```python
from build123d import *

# Parameters (mm, degrees)
F0_W     = 45
F0_H     = 45
F1_DEPTH = 3
F3_DEPTH = 25
F4_W     = 45
F4_H     = 45
F5_DEPTH = 5
F7_DEPTH = 25
F8_R     = 18
F9_DEPTH = 25


with BuildPart() as f1:
    # F0 (on Top) → F1 (new body)
    with BuildSketch(Plane.XY):
        Rectangle(F0_W, F0_H)
    extrude(amount=F1_DEPTH)

    # F2 (on face) → F3 (cut)
    with BuildSketch(Plane.XY.offset(3)):
        Polygon((11.5, 11.5), (-11.5, 11.5), (-11.5, 4), (-17.6846776158, 4), (-17.6846776158, -4), (-11.5, -4), (-11.5, -11.5), (11.5, -11.5), (11.5, -4), (17.6846776158, -4), (17.6846776158, 4), (11.5, 4), align=None)
    extrude(amount=-F3_DEPTH, mode=Mode.SUBTRACT)

    # F4 (on face) → F5 (join)
    with BuildSketch(Plane.XY.offset(3)):
        Rectangle(F4_W, F4_H)
    extrude(amount=F5_DEPTH)

    # F6 (on face) → F7 (cut)
    with BuildSketch(Plane(origin=(0, 0, 3), x_dir=(1, 0, 0), z_dir=(0, 0, -1))):
        Polygon((11.5, -11.5), (11.5, -4), (11.5, 4), (11.5, 11.5), (-11.5, 11.5), (-11.5, 4), (-11.5, -4), (-11.5, -11.5), align=None)
    extrude(amount=-F7_DEPTH, mode=Mode.SUBTRACT)

    # F8
    f8_edges = [f1.edges().sort_by_distance(p)[0] for p in [
        (-22.5, -22.5, 4),
        (22.5, -22.5, 4),
        (22.5, 22.5, 4),
        (-22.5, 22.5, 4),
    ]]
    fillet(f8_edges, radius=F8_R)

    # F9 (add): a face of the model
    f9_faces = [f1.faces().sort_by_distance(p)[0] for p in [
        (0, 21.8636038969, 8),
    ]]
    extrude(f9_faces, amount=F9_DEPTH)


solid = f1.part
```
Part model, mm, in its own coordinate system. A direction names the side the tool comes from. Round coordinates to 2 decimals unless told otherwise and drop trailing zeros. Write each loop counter-clockwise with the first axis right and the second up, starting at its lowest first coordinate (ties: lowest second). Pieces come first, ordered by that corner, then holes.
Item 1: Cut at D-D, the plane x = 17. Give the cut face in (y, z), plus the area to 3 significant figures.
Results:
outline: (-17.45, 0) - (-4, 0) - (-4, 3) - (4, 3) - (4, 0) - (17.45, 0) - (17.45, 33) - (-17.45, 33) - close
area: 1,130 mm2
Item 2: Which spindle directions (+Z, -Z, +X, -X, +Y, -Y) get a long thin tool onto all of the face, cutting with end or side? Do faces 4 (the flat face through (0, -15, 0)), 5 (the flat face through (-15, 0, 3)). Say none if no direction does.
Results:
face 4: -Z, +X, -X, +Y, -Y
face 5: -Z
Item 3: Cut at A-A, the plane x = -2.5. Give the cut face in (y, z), plus the area to 3 significant figures.
Results:
outline: (-22.5, 0) - (-11.5, 0) - (-11.5, 33) - (-22.5, 33) - close; (11.5, 0) - (22.5, 0) - (22.5, 33) - (11.5, 33) - close
area: 726 mm2
Item 4: Cut at B-B, the plane y = -1.5. Give the cut face in (x, z).
Results:
outline: (-22.5, 0) - (-17.68, 0) - (-17.68, 3) - (-11.5, 3) - (-11.5, 33) - (-22.5, 33) - close; (11.5, 3) - (17.68, 3) - (17.68, 0) - (22.5, 0) - (22.5, 33) - (11.5, 33) - close
Item 5: Cut at C-C, the plane z = 14. Give the cut face in (x, y).
Results:
outline: (-22.5, -4.5) arc R18 ccw to (-4.5, -22.5) - (4.5, -22.5) arc R18 ccw to (22.5, -4.5) - (22.5, 4.5) arc R18 ccw to (4.5, 22.5) - (-4.5, 22.5) arc R18 ccw to (-22.5, 4.5) - close; hole (-11.5, -11.5) - (11.5, -11.5) - (11.5, 11.5) - (-11.5, 11.5) - close
Item 6: Probe L1, parallel to X at y = -5, z = 16.5; L2, parallel to Y at x = -2, z = 20; L3, parallel to Y at x = -6, z = 18.5. List the from-to ranges inside material, lowest first.
Results:
L1: x = -22.49 to -11.5, 11.5 to 22.49
L2: y = -22.5 to -11.5, 11.5 to 22.5
L3: y = -22.44 to -11.5, 11.5 to 22.44
Item 7: Two-plate mould, pull along X, no slides. Class faces 1 (the flat face through (-22.5, 0, 16)), 2 (the flat face through (-15, -4, 2)), 3 (the flat face through (-15, 0, 33)): +X half, -X half, draft (parallel to the pull), parting line (faces both ways), or undercut.
Results:
face 1: -X half
face 2: undercut
face 3: draft
Item 8: Drop flat-ended pins along their axis: pin 1 Ø3 at (x, y) = (15.5, -2) entering from -Z; pin 2 Ø10 at (y, z) = (11.5, 9) entering from -X; pin 3 Ø1.5 at (x, z) = (6.5, 3.5) entering from -Y. Give the stop position or say it passes through.
Results:
pin 1: stops at z = 3
pin 2: stops at x = -22.39
pin 3: stops at y = -22.46
